Geometry check sheet. Reference: the model listing, model coordinates, mm. A direction names the side the tool comes from. Round coordinates to 2 decimals unless told otherwise and drop trailing zeros. Write each loop counter-clockwise with the first axis right and the second up, starting at its lowest first coordinate (ties: lowest second). Pieces come first, ordered by that corner, then holes. Notation, with made-up numbers: (-14.75, 28.5) -> (12.25, 28.5) arc R8 ccw to (12.25, 42.5) -> close; hole circle Ø2 at (-20.5, 26.5). An arc over 180 degrees is marked (long way). Return JSON: item names as keys, results as strings. Group by question number.
from build123d import *

# Parameters (mm, degrees)
CUT_EXTRUDE_1_DEPTH      = 5
CUT_EXTRUDE_1_DEPTH_BACK = 5
CUT_EXTRUDE_2_DEPTH      = 5
CUT_EXTRUDE_2_DEPTH_BACK = 5


with BuildPart() as part:
    # Sketch 1 → Revolve 1 (revolve)
    with BuildSketch(Plane.XY, mode=Mode.PRIVATE) as revolve_1_sk:
        Polygon((0, 0), (0, 4.233), (0.767, 5), (22, 5), (23, 6), (521, 6), (521, 15.75), (543, 15.75), (543, 0), align=None)
    revolve(revolve_1_sk.sketch.rotate(Axis((543, 0, 0), (-1, 0, 0)), 270), axis=Axis((543, 0, 0), (-1, 0, 0)))

    # Sketch 2 → Cut-Extrude 1 (cut, two sides: drawn at the far end of the back side and taken through both)
    with BuildSketch(Plane(origin=(0, 0, 0), x_dir=(1, 0, 0), z_dir=(0, -0.7071067811865477, 0.7071067811865475)).offset(-CUT_EXTRUDE_1_DEPTH_BACK)):
        Polygon((-5, -12), (35.4, -12), (28.4, -5), (22, -5), (19.8, -7.2), (19.8, -10), (-3, -10), (-3, 10), (19.8, 10), (19.8, 7.2), (22, 5), (28.4, 5), (35.4, 12), (-5, 12), align=None)
    extrude(amount=CUT_EXTRUDE_1_DEPTH + CUT_EXTRUDE_1_DEPTH_BACK, mode=Mode.SUBTRACT)

    # Sketch 3 → Cut-Extrude 2 (cut, two sides: drawn at the far end of the back side and taken through both)
    with BuildSketch(Plane(origin=(0, 0, 0), x_dir=(-1, 0, 0), z_dir=(0, -0.7071067811865477, -0.7071067811865475)).offset(-CUT_EXTRUDE_2_DEPTH_BACK)):
        Polygon((5, 12), (-35.4, 12), (-28.4, 5), (-22, 5), (-19.8, 7.2), (-19.8, 10), (3, 10), (3, -10), (-19.8, -10), (-19.8, -7.2), (-22, -5), (-28.4, -5), (-35.4, -12), (5, -12), align=None)
    extrude(amount=CUT_EXTRUDE_2_DEPTH + CUT_EXTRUDE_2_DEPTH_BACK, mode=Mode.SUBTRACT)


solid = part.part
1) Tool access check on faces 1 (the face through (521, 0, -7)), 2 (the face through (0, 0, 0)). Record the directions out of +Z, -Z, +X, -X, +Y, -Y that give a thin tool (end or side, any length) a straight path to the whole face; none if there is none.
2) Material ranges on probe 1 along X at (y, z) = (-7.5, -2.5); probe 2 along Y at (x, z) = (259, 1); probe 3 along Z at (x, y) = (108.5, 3.5), recorded low to high. Write a range as [from, to].
3) Go/stop test with flat-tipped pins: P1, Ø10, axis at y = 11.5, z = 5.5, coming from the -X side; P2, Ø6, axis at x = 231.5, z = -7.5, coming from the +Y side; P3, Ø6, axis at y = 3.5, z = -7, coming from the -X side. Record where each tip stops, or that it passes through.
4) Sectioned sample at A-A on x = 101. Enter the section's corners in (y, z), and give its area (3 significant figures).
Evaluation:
{
 "1": {"face 1": "-X", "face 2": "+Z, -Z, -X, +Y, -Y"},
 "2": {"probe 1": "x = [521, 543]", "probe 2": "y = [-5.92, 5.92]", "probe 3": "z = [-4.87, 4.87]"},
 "3": {"P1": "stops at x = 521", "P2": "stops at y = 3.97", "P3": "stops at x = 0.59"},
 "4": {"outline": "circle Ø12 at (0, 0)", "area": "113 mm2"}
}
